```python
from build123d import *

# Parameters (mm, degrees)
SKETCH_1_R      = 2
EXTRUDE_1_DEPTH = 2.5


with BuildPart() as part:
    # 草圖1 → 填料-伸長1 (new, symmetric)
    with BuildSketch(Plane.XY):
        with BuildLine():
            Line((-21, -35), (21, -35))
            ThreePointArc((21, -35), (23.828427125, -33.828427125), (25, -31))
            Line((25, -31), (25, 31))
            ThreePointArc((25, 31), (23.828427125, 33.828427125), (21, 35))
            Line((21, 35), (-21, 35))
            ThreePointArc((-21, 35), (-23.828427125, 33.828427125), (-25, 31))
            Line((-25, 31), (-25, 7.788457268))
            ThreePointArc((-25, 7.788457268), (-25.535898385, 5.788457268), (-27, 4.324355653))
            Line((-27, 4.324355653), (-40.5, -3.469872981))
            ThreePointArc((-40.5, -3.469872981), (-42.330127019, -10.3), (-35.5, -12.130127019))
            Line((-35.5, -12.130127019), (-31, -9.532050808))
            ThreePointArc((-31, -9.532050808), (-27, -9.532050808), (-25, -12.996152423))
            Line((-25, -12.996152423), (-25, -31))
            ThreePointArc((-25, -31), (-23.828427125, -33.828427125), (-21, -35))
        make_face()
        Circle(SKETCH_1_R, mode=Mode.SUBTRACT)
        with Locations((-38, -7.8)):
            Circle(SKETCH_1_R, mode=Mode.SUBTRACT)
    extrude(amount=EXTRUDE_1_DEPTH, both=True)


solid = part.part
```
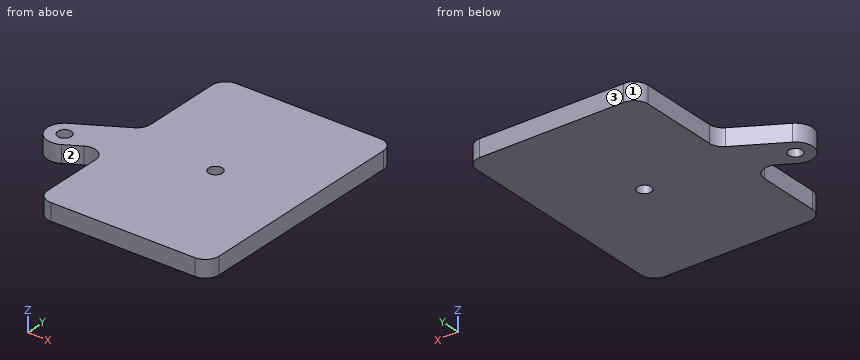
Could you check a few things on this model? Use its own coordinates, in mm. Face numbers are marked on the shaded views. Round coordinates to 2 decimals unless told otherwise and drop trailing zeros. Loops run counter-clockwise (first coordinate to the right, second up) from the corner with the lowest first, then second, coordinate; pieces in that order, holes last. Notation, with made-up numbers: (-27, 61.25) -> (-3, 61.25) arc R13 cw to (-3, 81.25) -> close; hole circle Ø11 at (-30.5, -39.5). An arc over 180 degrees is marked (long way). One line per question, with ' | ' between items.
(1) If we section it at C-C on z = 0.95: List the corners of the cut face in (x, y) for me, and give its area (3 significant figures).
Model answer:
outline: (-40.5, -3.47) arc R5 ccw to (-35.5, -12.13) -> (-31, -9.53) arc R4 cw to (-25, -13) -> (-25, -31) arc R4 ccw to (-21, -35) -> (21, -35) arc R4 ccw to (25, -31) -> (25, 31) arc R4 ccw to (21, 35) -> (-21, 35) arc R4 ccw to (-25, 31) -> (-25, 7.79) arc R4 cw to (-27, 4.32) -> close; hole circle Ø4 at (-38, -7.8); hole circle Ø4 at (0, 0) | area: 3,660 mm^2
(2) For pin 1 Ø1.5 at (y, z) = (-27, -1) entering from -X; pin 2 Ø2.5 at (x, y) = (0, 0) entering from +Z; pin 3 Ø2 at (y, z) = (4, -1.5) entering from -X, each with a flat end and sliding along its axis, tell me the tip position at first contact or that it passes through.
Model answer:
pin 1: stops at x = -25 | pin 2: passes through | pin 3: stops at x = -29.29
(3) If we section it at D-D on y = 21.5: List the corners of the cut face in (x, z) for me, and give its area (3 significant figures).
Model answer:
outline: (-25, -2.5) -> (25, -2.5) -> (25, 2.5) -> (-25, 2.5) -> close | area: 250 mm^2
(4) If we section it at B-B on x = 0: List the corners of the cut face in (y, z) for me.
Model answer:
outline: (-35, -2.5) -> (-2, -2.5) -> (-2, 2.5) -> (-35, 2.5) -> close; (2, -2.5) -> (35, -2.5) -> (35, 2.5) -> (2, 2.5) -> close
(5) If we section it at A-A on y = 0: List the corners of the cut face in (x, z) for me.
Model answer:
outline: (-34.49, -2.5) -> (-2, -2.5) -> (-2, 2.5) -> (-34.49, 2.5) -> close; (2, -2.5) -> (25, -2.5) -> (25, 2.5) -> (2, 2.5) -> close
(6) If I drill on probe 1 along Y at (x, z) = (0, -0.65); probe 2 along Y at (x, z) = (-38, -0.05); probe 3 along X at (y, z) = (-29, -2), over which ranges is the centre line in solid material (lowest first)?
Model answer:
probe 1: y = -35 to -2, 2 to 35 | probe 2: y = -12.8 to -9.8, -5.8 to -2.03 | probe 3: x = -25 to 25
(7) Thinking about a two-plate mould opening in X: for the marked faces 1, 2 and 3, which applies, released by +X, released by -X, zero draft, split by the parting line, or undercut?
Model answer:
face 1: released by -X | face 2: undercut | face 3: zero draft
